Answer from the drawing. Dimensions are ordinates in mm from the lowest x, y and z of the part. A direction names the side the tool comes from. Coordinates: 2 decimals unless noted, no trailing zeros. Write each loop counter-clockwise with the first axis right and the second up, starting at its lowest first coordinate (ties: lowest second). Pieces come first, ordered by that corner, then holes.
1) The part is cut by section A-A (z = 2.5). Determine the outline of the cut face in (x, y).
2) The part is cut by section D-D (z = 4.2). Determine the outline of the cut face in (x, y).
3) Which of the six approach directions +Z, -Z, +X, -X, +Y, -Y give full straight-line access (tool end or side, diameter ignored) to the marked faces 1 and 2?
4) This flat-tipped pin is pushed along its axis until it touches: pin 1 Ø2 at (x, z) = (6, 2) entering from +Y. Where does it stop, or does it pass through?
5) The part is cut by section C-C (y = 9.25). Determine the outline of the cut face in (x, z).
6) Find the intervals of material crossed by line 1 (Z direction, x = 6.5, y = 5.25); line 2 (X direction, y = 9.65, z = 2.5); line 3 (Z direction, x = 6.5, y = 9.15), in increasing order.
7) The part is cut by section B-B (x = 6.5). Determine the outline of the cut face in (y, z).
8) Determine the mould class of the marked faces 3, 4 and 5 for opening direction Z: +Z half, -Z half, draft (parallel to the pull), parting line (faces both ways), or undercut.
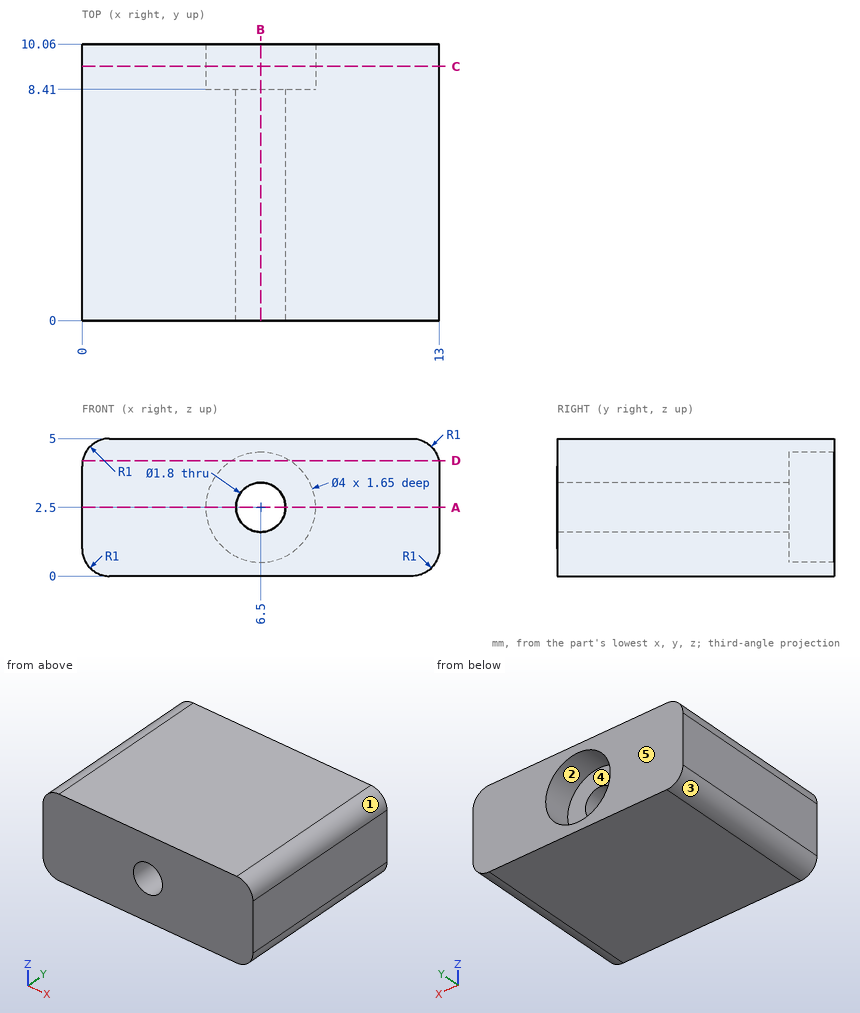
Reported:
1. outline: (0, 0) - (5.6, 0) - (5.6, 8.41) - (4.5, 8.41) - (4.5, 10.06) - (0, 10.06) - close; (7.4, 0) - (13, 0) - (13, 10.06) - (8.5, 10.06) - (8.5, 8.41) - (7.4, 8.41) - close
2. outline: (0.02, 0) - (12.98, 0) - (12.98, 10.06) - (7.55, 10.06) - (7.55, 8.41) - (5.45, 8.41) - (5.45, 10.06) - (0.02, 10.06) - close
3. face 1: +Z, +X, +Y, -Y
3. face 2: +Y
4. pin 1: stops at y = 8.41
5. outline: (0, 1) arc R1 ccw to (1, 0) - (12, 0) arc R1 ccw to (13, 1) - (13, 4) arc R1 ccw to (12, 5) - (1, 5) arc R1 ccw to (0, 4) - close; hole circle Ø4 at (6.5, 2.5)
6. line 1: z = 0 to 1.6, 3.4 to 5
6. line 2: x = 0 to 4.5, 8.5 to 13
6. line 3: z = 0 to 0.5, 4.5 to 5
7. outline: (0, 0) - (10.06, 0) - (10.06, 0.5) - (8.41, 0.5) - (8.41, 1.6) - (0, 1.6) - close; (0, 3.4) - (8.41, 3.4) - (8.41, 4.5) - (10.06, 4.5) - (10.06, 5) - (0, 5) - close
8. face 3: -Z half
8. face 4: undercut
8. face 5: draft
